Here's how the part is built. I have some questions about the finished solid (model axes, mm). Round coordinates to 2 decimals unless told otherwise and drop trailing zeros. Write each loop counter-clockwise with the first axis right and the second up, starting at its lowest first coordinate (ties: lowest second). Pieces come first, ordered by that corner, then holes. Notation, with made-up numbers: (79.25, 64.5) - (124.25, 64.5) arc R11 ccw to (124.25, 81.5) - close; hole circle Ø3 at (44.25, -39.75). An arc over 180 degrees is marked (long way). Write item = value, one per line. Start each with the question number.
Item 1: If we section it at B-B (z = 0): Please give me the cut outline in (x, y) (3 decimals).
Item 2: For P1, Ø1, axis at y = 14.5, z = 1.5, coming from the -X side; P2, Ø2, axis at x = 1.5, z = 0, coming from the +Y side, each with a flat end and sliding along its axis, tell me the tip position at first contact or that it passes through.
Item 3: If we section it at D-D (z = 1): Please give me the cut outline in (x, y) (1 decimal).
Item 4: If we section it at C-C (y = 2.5): Please give me the cut outline in (x, z), and give its area (3 significant figures).
Item 5: If I drill on line 1 along Y through (x, z) = (-1.6, -1.55) (3 decimals); line 2 along Z through (x, y) = (-0.6, 3.5); line 3 along Z through (x, y) = (1.45, 16), over which ranges is the centre line in solid material (lowest first)? Write a range as [from, to].
Item 6: If we section it at A-A (x = 0): Please give me the cut outline in (y, z) (3 decimals).
Item 7: Thinking about a two-plate mould opening in X: for faces 1 (the face through (1.6, 13.44, 0.83)), 2 (the face through (0, 0.787, 0)), 3 (the face through (2, 9.525, 1)), which applies, pulls with the +X half, pulls with the -X half, needs draft (parallel to the pull), parting line crosses it, or undercut?
```python
from build123d import *

# Parameters (mm, degrees)
CUT_EXTRUDE1_DEPTH      = 20.441008011
CUT_EXTRUDE1_DEPTH_BACK = 20.441008011
SKETCH2_W               = 1.1684
SKETCH2_H               = 0.7874


with BuildPart() as part:
    # Sketch1 → Revolve1 (revolve)
    with BuildSketch(Plane.XY, mode=Mode.PRIVATE) as revolve1_sk:
        with BuildLine():
            Line((0, 19.05), (0, 0))
            Line((0, 0), (2.7432, 0))
            Line((2.7432, 0), (2.7432, 9.525))
            Line((2.7432, 9.525), (1.8034, 9.525))
            Line((1.8034, 9.525), (1.8034, 17.2466))
            ThreePointArc((1.8034, 17.2466), (1.275196369, 18.521796369), (0, 19.05))
        make_face()
    revolve(revolve1_sk.sketch.rotate(Axis((0, 19.05, 0), (0, -1, 0)), 90), axis=Axis((0, 19.05, 0), (0, -1, 0)))

    # Sketch2 → Cut-Extrude1 (cut, two sides: drawn at the far end of the back side and taken through both)
    with BuildSketch(Plane.XY.offset(-CUT_EXTRUDE1_DEPTH_BACK)):
        with Locations((0, 0.3937)):
            Rectangle(SKETCH2_W, SKETCH2_H)
    extrude(amount=CUT_EXTRUDE1_DEPTH + CUT_EXTRUDE1_DEPTH_BACK, mode=Mode.SUBTRACT)


solid = part.part
```
Reply:
q1.outline = (-2.743, 0) - (-0.584, 0) - (-0.584, 0.787) - (0.584, 0.787) - (0.584, 0) - (2.743, 0) - (2.743, 9.525) - (1.803, 9.525) - (1.803, 17.247) arc R1.803 ccw to (-1.803, 17.247) - (-1.803, 9.525) - (-2.743, 9.525) - close
q2.P1 = -1.5
q2.P2 = 18.98
q3.outline = (-2.6, 0) - (-0.6, 0) - (-0.6, 0.8) - (0.6, 0.8) - (0.6, 0) - (2.6, 0) - (2.6, 9.5) - (1.5, 9.5) - (1.5, 17.2) arc R1.5 ccw to (-1.5, 17.2) - (-1.5, 9.5) - (-2.6, 9.5) - close
q4.outline = circle Ø5.49 at (0, 0)
q4.area = 23.6 mm2
q5.line_1 = [0, 9.525]
q5.line_2 = [-2.68, 2.68]
q5.line_3 = [-1.07, 1.07]
q6.outline = (0.787, -2.743) - (9.525, -2.743) - (9.525, -1.803) - (17.247, -1.803) arc R1.803 ccw to (17.247, 1.803) - (9.525, 1.803) - (9.525, 2.743) - (0.787, 2.743) - close
q7.face_1 = parting line crosses it
q7.face_2 = undercut
q7.face_3 = needs draft
